```python
from build123d import *

# Parameters (mm, degrees)
ESQUISSE1_W             = 43
ESQUISSE1_H             = 36
BOSS_EXTRU_1_DEPTH      = 3
ESQUISSE2_W             = 3
ESQUISSE2_H             = 36
BOSS_EXTRU_2_DEPTH      = 25
ESQUISSE3_W             = 3
ESQUISSE3_H             = 36
BOSS_EXTRU_3_DEPTH      = 35
ESQUISSE4_R             = 2.5
ENL_V_MAT_EXTRU_1_DEPTH = 95
CONG_1_R                = 20
ESQUISSE5_W             = 46.070025289
ESQUISSE5_H             = 43.599493682
ENL_V_MAT_EXTRU_2_DEPTH = 95
ESQUISSE6_W             = 3
ESQUISSE6_H             = 36
BOSS_EXTRU_4_DEPTH      = 35
ESQUISSE7_R             = 2.482615241
ENL_V_MAT_EXTRU_3_DEPTH = 35
CONG_2_R                = 20


with BuildPart() as part:
    # Esquisse1 → Boss.-Extru.1 (new body)
    with BuildSketch(Plane.XY):
        with Locations((-52.514246193, 13.599576988)):
            Rectangle(ESQUISSE1_W, ESQUISSE1_H)
    extrude(amount=BOSS_EXTRU_1_DEPTH)

    # Esquisse2 → Boss.-Extru.2 (add)
    with BuildSketch(Plane.XY.offset(3)):
        with Locations((-32.514246193, 13.599576988)):
            Rectangle(ESQUISSE2_W, ESQUISSE2_H)
    extrude(amount=BOSS_EXTRU_2_DEPTH)

    # Esquisse3 → Boss.-Extru.3 (add)
    with BuildSketch(Plane.XY.offset(3)):
        with Locations((-72.514246193, 13.599576988)):
            Rectangle(ESQUISSE3_W, ESQUISSE3_H)
    extrude(amount=BOSS_EXTRU_3_DEPTH)

    # Esquisse4 → Enlèv. mat.-Extru.1 (cut)
    with BuildSketch(Plane.ZY.offset(74.014246193)):
        with Locations(Location((31, 14.099576988, 0), (0, 0, 270))):
            Circle(ESQUISSE4_R)
    extrude(amount=-ENL_V_MAT_EXTRU_1_DEPTH, mode=Mode.SUBTRACT)

    # Congé1
    # the kernel refuses this fillet: 20 mm, written as the material it takes off along each edge
    with BuildSketch(Plane(origin=(-34.014246193, -4.400423012, 28), x_dir=(0, 1, 0), z_dir=(1, 0, 0))) as cong_1_piece_1:
        with BuildLine():
            CenterArc((CONG_1_R, -CONG_1_R), CONG_1_R, 90, 90)
            Line((0, -CONG_1_R), (0, 0))
            Line((0, 0), (CONG_1_R, 0))
        make_face()
    extrude(amount=53, mode=Mode.SUBTRACT)
    with BuildSketch(Plane(origin=(18.985753807, 31.599576988, 28), x_dir=(0, 0, -1), z_dir=(-1, 0, 0))) as cong_1_piece_2:
        with BuildLine():
            CenterArc((CONG_1_R, CONG_1_R), CONG_1_R, 180, 90)
            Line((0, CONG_1_R), (0, 0))
            Line((0, 0), (CONG_1_R, 0))
        make_face()
    extrude(amount=53, mode=Mode.SUBTRACT)
    with BuildSketch(Plane(origin=(-21.014246193, -4.400423012, 38), x_dir=(0, 1, 0), z_dir=(-1, 0, 0))) as cong_1_piece_3:
        with BuildLine():
            CenterArc((CONG_1_R, CONG_1_R), CONG_1_R, 180, 90)
            Line((0, CONG_1_R), (0, 0))
            Line((0, 0), (CONG_1_R, 0))
        make_face()
    extrude(amount=103, mode=Mode.SUBTRACT)
    with BuildSketch(Plane(origin=(-124.014246193, 31.599576988, 38), x_dir=(0, 0, -1), z_dir=(1, 0, 0))) as cong_1_piece_4:
        with BuildLine():
            CenterArc((CONG_1_R, -CONG_1_R), CONG_1_R, 90, 90)
            Line((0, -CONG_1_R), (0, 0))
            Line((0, 0), (CONG_1_R, 0))
        make_face()
    extrude(amount=103, mode=Mode.SUBTRACT)

    # Esquisse5 → Enlèv. mat.-Extru.2 (cut)
    with BuildSketch(Plane.ZY.offset(34.014246193)):
        with Locations((26.035012645, 9.799830147)):
            Rectangle(ESQUISSE5_W, ESQUISSE5_H)
    extrude(amount=-ENL_V_MAT_EXTRU_2_DEPTH, mode=Mode.SUBTRACT)

    # Esquisse6 → Boss.-Extru.4 (add)
    with BuildSketch(Plane.XY.offset(3)):
        with Locations((-32.514246193, 13.599576988)):
            Rectangle(ESQUISSE6_W, ESQUISSE6_H)
    extrude(amount=BOSS_EXTRU_4_DEPTH)

    # Esquisse7 → Enlèv. mat.-Extru.3 (cut)
    with BuildSketch(Plane.ZY.offset(34.014246193)):
        with Locations((30.985935606, 14.217034277)):
            Circle(ESQUISSE7_R)
    extrude(amount=-ENL_V_MAT_EXTRU_3_DEPTH, mode=Mode.SUBTRACT)

    # Congé2
    # the kernel refuses this fillet: 20 mm, written as the material it takes off along each edge
    with BuildSketch(Plane(origin=(-84.014246193, -4.400423012, 38), x_dir=(0, 1, 0), z_dir=(1, 0, 0))) as cong_2_piece_1:
        with BuildLine():
            CenterArc((CONG_2_R, -CONG_2_R), CONG_2_R, 90, 90)
            Line((0, -CONG_2_R), (0, 0))
            Line((0, 0), (CONG_2_R, 0))
        make_face()
    extrude(amount=103, mode=Mode.SUBTRACT)
    with BuildSketch(Plane(origin=(18.985753807, 31.599576988, 38), x_dir=(0, 0, -1), z_dir=(-1, 0, 0))) as cong_2_piece_2:
        with BuildLine():
            CenterArc((CONG_2_R, CONG_2_R), CONG_2_R, 180, 90)
            Line((0, CONG_2_R), (0, 0))
            Line((0, 0), (CONG_2_R, 0))
        make_face()
    extrude(amount=103, mode=Mode.SUBTRACT)


solid = part.part
```
Geometry check sheet. Reference: the model listing, model coordinates, mm. A direction names the side the tool comes from. Coordinates: 2 decimals unless noted, no trailing zeros. Order: outer loops, then holes, each group sorted by start corner. A loop starts at its lowest first (then second) coordinate and runs counter-clockwise, first axis right, second up. Notation, with made-up numbers: (46.5, 53.25) - (91.5, 53.25) arc R35 ccw to (91.5, 92.25) - close; hole circle Ø11 at (45, 4). An arc over 180 degrees is marked (long way). Answer as a JSON object with one key per item and string values. Group by question number.
Item 1: Sectioned sample at D-D, the plane x = -54.5. Record the cut outline in (y, z).
Item 2: Sectioned sample at C-C, the plane y = 20.5. Record the cut outline in (x, z).
Item 3: Sectioned sample at B-B, the plane z = 31. Record the cut outline in (x, y), and give its area (3 significant figures).
Item 4: Depth check by flat-ended pin: pin 1 Ø3 at (y, z) = (14.1, 31) entering from +X; pin 2 Ø10 at (x, y) = (-47, 8) entering from +Z. Enter the tip coordinate at first touch or a pass-through.
Item 5: Scan lines: probe 1 along X at (y, z) = (11.5, 34.5); probe 2 along Z at (x, y) = (-64, 2.5). Record each from-to range of solid material in increasing order.
Item 6: Draft check along Y on faces 4 (the face through (-32.535, 14.326, 28.506)), 5 (the face through (-72.493, 0.63, 31.263)), 6 (the face through (-34.014, 13, 16)). Enter one of: +Y half, -Y half, draft (parallel to the pull), parting line (faces both ways), or undercut.
Item 7: Tool access check on faces 1 (the face through (-72.54, 15.94, 32.69)), 2 (the face through (-53, 13, 3)), 3 (the face through (-53, 31.6, 1)). Record the directions out of +Z, -Z, +X, -X, +Y, -Y that give a thin tool (end or side, any length) a straight path to the whole face; none if there is none.
Item 8: Sectioned sample at A-A, the plane z = 11. Record the cut outline in (x, y).
Resolved:
{
 "1": {"outline": "(-4.4, 0) - (31.6, 0) - (31.6, 3) - (-4.4, 3) - close"},
 "2": {"outline": "(-74.01, 0) - (-31.01, 0) - (-31.01, 35.91) - (-34.01, 35.91) - (-34.01, 3) - (-71.01, 3) - (-71.01, 35.91) - (-74.01, 35.91) - close"},
 "3": {"outline": "(-74.01, 0.4) - (-71.01, 0.4) - (-71.01, 11.6) - (-74.01, 11.6) - close; (-74.01, 16.6) - (-71.01, 16.6) - (-71.01, 26.8) - (-74.01, 26.8) - close; (-34.01, 0.4) - (-31.01, 0.4) - (-31.01, 11.73) - (-34.01, 11.73) - close; (-34.01, 16.7) - (-31.01, 16.7) - (-31.01, 26.8) - (-34.01, 26.8) - close", "area": "128 mm^2"},
 "4": {"pin 1": "through", "pin 2": "z = 3"},
 "5": {"probe 1": "-74.01 to -71.01, -34.01 to -31.01", "probe 2": "0 to 3"},
 "6": {"face 4": "undercut", "face 5": "-Y half", "face 6": "draft"},
 "7": {"face 1": "-X", "face 2": "+Z, +Y, -Y", "face 3": "+Z, -Z, +X, -X, +Y"},
 "8": {"outline": "(-74.01, -4.4) - (-71.01, -4.4) - (-71.01, 31.6) - (-74.01, 31.6) - close; (-34.01, -4.4) - (-31.01, -4.4) - (-31.01, 31.6) - (-34.01, 31.6) - close"}
}
